Autodesk Inventor part; units mm, degrees
ref_plane "YZ Plane" through (0, 0, 0) normal (1, 0, 0) x (0, 1, 0)
ref_plane "XZ Plane" through (0, 0, 0) normal (0, 1, 0) x (-1, 0, 0)
ref_plane "XY Plane" through (0, 0, 0) normal (0, 0, 1) x (1, 0, 0)
sketch "Szkic1" plane through (0, 0, 0) normal (0, 1, 0) x (-1, 0, 0)
  circle A0 centre (0, 0) radius 15
  dimension "d0" = 30
extrude "Wyciągnięcie proste1" add sketch "Szkic1" along normal blind 2
sketch "Szkic2" plane through (0, 2, 0) normal (0, 1, 0) x (1, 0, 0)
  circle A0 centre (0, 0) radius 12.5
  dimension "d3" = 25
extrude "Wyciągnięcie proste2" add sketch "Szkic2" along normal blind 4
sketch "Szkic9" plane through (0, 6, 0) normal (0, 1, 0) x (1, 0, 0)
  circle A0 centre (0, 0) radius 12
  dimension "d22" = 24
extrude "Wyciągnięcie proste7" add sketch "Szkic9" along normal blind 2
sketch "Szkic11" plane through (0, 8, 0) normal (0, 1, 0) x (1, 0, 0)
  circle A0 centre (1.5, -6) radius 1.45
  circle A1 centre (1.5, 6) radius 1.45
  point P0 (0, 0)
  dimension "d25" = 2.9
  dimension "d26" = 2.9
extrude "Wyciągnięcie proste8" cut sketch "Szkic11" against normal blind 6
sketch "Szkic5" plane through (0, 0, 0) normal (0, -1, 0) x (1, 0, 0)
  arc A0 (-0.62, -1.59) -> (-0.62, 1.59) centre (1.5, 0) ccw
  line L0 (-0.62, 1.59) -> (-0.62, -1.59)
  point P0 (0, 0)
extrude "Wyciągnięcie proste5" cut sketch "Szkic5" against normal blind 8
properties part number "Rotor_shaft_21"
Input: part model. Units: mm. Frame: model coordinates. A direction names the side the tool comes from. Round coordinates to 2 decimals unless told otherwise and drop trailing zeros. Order: outer loops, then holes, each group sorted by start corner. A loop starts at its lowest first (then second) coordinate and runs counter-clockwise, first axis right, second up. Notation, with made-up numbers: (68, 63) - (119, 63) arc R9 cw to (119, 73) - close; hole circle Ø7 at (-17, 67.5). An arc over 180 degrees is marked (long way). Answer in a Markdown table with one row per item.
Item 1: Section query D-D (x = -1.5). Return the cut outline in (y, z), then the cut area to 3 significant figures.
Model answer:
| item | result |
|---|---|
| outline | (0, -14.92) - (2, -14.92) - (2, -12.41) - (6, -12.41) - (6, -11.91) - (8, -11.91) - (8, 11.91) - (6, 11.91) - (6, 12.41) - (2, 12.41) - (2, 14.92) - (0, 14.92) - close |
| area | 207 mm² |
Item 2: Line query: line 1 (Z direction, x = 1.5, y = 4.1); line 2 (Z direction, x = 2, y = 7.25); line 3 (X direction, y = 4.5, z = 3.5). Output: solid intervals per line, ascending.
Model answer:
| item | result |
|---|---|
| line 1 | z = -12.41 to -7.45, -4.55 to -2.65, 2.65 to 4.55, 7.45 to 12.41 |
| line 2 | z = -11.83 to -7.36, -4.64 to -2.6, 2.6 to 4.64, 7.36 to 11.83 |
| line 3 | x = -12 to 12 |
Item 3: Reachability of faces 1 (the cylindrical face through (-11.99, 6.99, 0.53)), 2 (the flat face through (-0.62, 4, 0)), 3 (the flat face through (-3, 0, 0)) from +Z, -Z, +X, -X, +Y, -Y: full face, straight path, thin tool, end or side. Return the list, or none.
Model answer:
| item | result |
|---|---|
| face 1 | +Y |
| face 2 | +Y, -Y |
| face 3 | +Z, -Z, +X, -X, -Y |
Item 4: Section query A-A (z = 0). Return the cut outline in (x, y).
Model answer:
| item | result |
|---|---|
| outline | (-15, 0) - (-0.62, 0) - (-0.62, 8) - (-12, 8) - (-12, 6) - (-12.5, 6) - (-12.5, 2) - (-15, 2) - close; (4.15, 0) - (15, 0) - (15, 2) - (12.5, 2) - (12.5, 6) - (12, 6) - (12, 8) - (4.15, 8) - close |
Item 5: Section query B-B (y = 7). Return the cut outline in (x, z), then the cut area to 3 significant figures.
Model answer:
| item | result |
|---|---|
| outline | circle Ø24 at (0, 0); hole (-0.62, -1.59) arc R2.65 ccw (long way) to (-0.62, 1.59) - close; hole circle Ø2.9 at (1.5, -6); hole circle Ø2.9 at (1.5, 6) |
| area | 418 mm² |
Item 6: Section query C-C (x = 1.5). Return the cut outline in (y, z), then the cut area to 3 significant figures.
Model answer:
| item | result |
|---|---|
| outline | (0, -14.92) - (2, -14.92) - (2, -12.41) - (6, -12.41) - (6, -11.91) - (8, -11.91) - (8, -7.45) - (2, -7.45) - (2, -4.55) - (8, -4.55) - (8, -2.65) - (0, -2.65) - close; (0, 2.65) - (8, 2.65) - (8, 4.55) - (2, 4.55) - (2, 7.45) - (8, 7.45) - (8, 11.91) - (6, 11.91) - (6, 12.41) - (2, 12.41) - (2, 14.92) - (0, 14.92) - close |
| area | 129 mm² |
Item 7: Pin query (flat end, axial travel): pin 1 (3 mm diameter, centred on y = 1, z = -6, fed in from +X); pin 2 (2.5 mm diameter, centred on x = 1.5, z = 6, fed in from +Y). Return the tip coordinate at first contact, or that it passes through.
Model answer:
| item | result |
|---|---|
| pin 1 | stops at x = 14.31 |
| pin 2 | stops at y = 2 |
Item 8: Mould query, pull axis X, two halves, no side actions, for faces 4 (the flat face through (1, 2, 6)), 5 (the cylindrical face through (2.28, 5.04, -7.22)), 6 (the flat face through (-0.2, 8, 2.5)), 7 (the cylindrical face through (14.985, 0.986, -0.66)). Classes: released by +X, released by -X, zero draft, split by the parting line, or undercut.
Model answer:
| item | result |
|---|---|
| face 4 | undercut |
| face 5 | undercut |
| face 6 | zero draft |
| face 7 | split by the parting line |
